```python
from build123d import *

# Parameters (mm, degrees)
BOSS_EXTRUDE1_DEPTH = 3
SKETCH2_R           = 1.5
SKETCH2_R_2         = 1.75
CUT_EXTRUDE1_DEPTH  = 131.896905999
SKETCH3_R           = 1.5
SKETCH3_W           = 5
SKETCH3_H           = 5
CUT_EXTRUDE2_DEPTH  = 131.896905999


with BuildPart() as part:
    # Sketch1 → Boss-Extrude1 (new body)
    with BuildSketch(Plane.XY):
        Polygon((0, 0), (3, 0), (3, -5), (50, -5), (50, -2), (80, -2), (80, -5), (127, -5), (127, 0), (130, 0), (130, 10), (127, 10), (127, 15), (3, 15), (3, 10), (0, 10), align=None)
    extrude(amount=BOSS_EXTRUDE1_DEPTH)

    # Sketch2 → Cut-Extrude1 (cut, through all)
    with BuildSketch(Plane.XY.offset(3)):
        with Locations((15, 8)):
            Circle(SKETCH2_R)
        with Locations((15, -2)):
            Circle(SKETCH2_R)
        with Locations((6, 8)):
            Circle(SKETCH2_R_2)
    extrude(amount=-CUT_EXTRUDE1_DEPTH, mode=Mode.SUBTRACT)

    # Sketch3 → Cut-Extrude2 (cut, through all)
    with BuildSketch(Plane.XY.offset(3)):
        with Locations((49, 7)):
            Circle(SKETCH3_R)
        with Locations((81, 7)):
            Circle(SKETCH3_R)
        with Locations((56.5, 7)):
            Rectangle(SKETCH3_W, SKETCH3_H)
    extrude(amount=-CUT_EXTRUDE2_DEPTH, mode=Mode.SUBTRACT)


solid = part.part
```
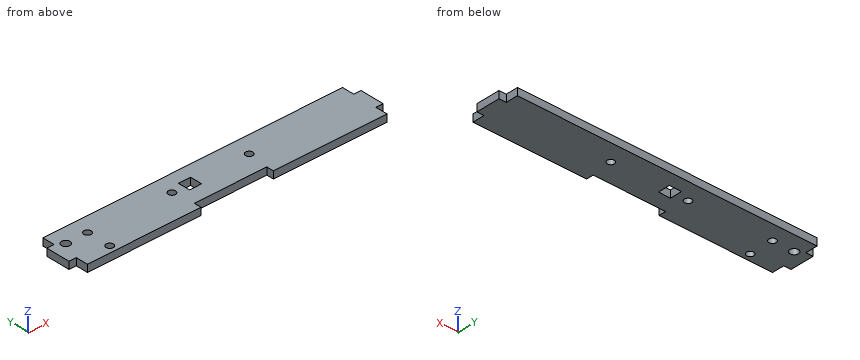
Can you work these out from the model? Positions are in its coordinate system, mm. Round coordinates to 2 decimals unless told otherwise and drop trailing zeros. Order: outer loops, then holes, each group sorted by start corner. A loop starts at its lowest first (then second) coordinate and runs counter-clockwise, first axis right, second up.
(1) If I drill on L1, parallel to Y at x = 15, z = 0.55; L2, parallel to X at y = 5.25, z = 1; L3, parallel to Y at x = 81, z = 0.9, over which ranges is the centre line in solid material (lowest first)?
Results are:
L1: y = -5 to -3.5, -0.5 to 6.5, 9.5 to 15
L2: x = 0 to 54, 59 to 130
L3: y = -5 to 5.5, 8.5 to 15
(2) If we section it at A-A (x = 15): Please give me the cut outline in (y, z).
Results are:
outline: (-5, 0) - (-3.5, 0) - (-3.5, 3) - (-5, 3) - close; (-0.5, 0) - (6.5, 0) - (6.5, 3) - (-0.5, 3) - close; (9.5, 0) - (15, 0) - (15, 3) - (9.5, 3) - close
(3) If we section it at B-B (z = 0.9): Please give me the cut outline in (x, y).
Results are:
outline: (0, 0) - (3, 0) - (3, -5) - (50, -5) - (50, -2) - (80, -2) - (80, -5) - (127, -5) - (127, 0) - (130, 0) - (130, 10) - (127, 10) - (127, 15) - (3, 15) - (3, 10) - (0, 10) - close; hole circle Ø3.5 at (6, 8); hole circle Ø3 at (15, -2); hole circle Ø3 at (15, 8); hole circle Ø3 at (49, 7); hole (54, 4.5) - (59, 4.5) - (59, 9.5) - (54, 9.5) - close; hole circle Ø3 at (81, 7)
(4) I'm going to push flat-ended pins straight in: pin 1 (0.9 mm diameter, centred on y = -3.5, z = 1.5, fed in from -X); pin 2 (1.5 mm diameter, centred on x = 128, z = 2, fed in from +Y); pin 3 (1.8 mm diameter, centred on x = 15, y = -2, fed in from +Z). Where does each tip first touch, or does it pass through?
Results are:
pin 1: stops at x = 3
pin 2: stops at y = 10
pin 3: passes through
